from build123d import *

# Parameters (mm, degrees)
EXTRUDE_1_DEPTH     = 3
SKETCH_2_R          = 1.65
CUT_EXTRUDE_1_DEPTH = 10
SKETCH_3_R          = 1.65
CUT_EXTRUDE_2_DEPTH = 10
SKETCH_4_R          = 1.65
CUT_EXTRUDE_3_DEPTH = 10
SKETCH_5_R          = 1.65
CUT_EXTRUDE_4_DEPTH = 10
SKETCH_6_R          = 1.65
CUT_EXTRUDE_5_DEPTH = 10
SKETCH_7_R          = 1.65
CUT_EXTRUDE_6_DEPTH = 10
CUT_EXTRUDE_7_DEPTH = 10
FILLET_1_R          = 5


with BuildPart() as part:
    # 草图1 → 凸台-拉伸1 (new body)
    with BuildSketch(Plane.XY):
        with BuildLine():
            Line((-87.5, 103.859649123), (87.5, 103.859649123))
            ThreePointArc((87.5, 103.859649123), (91.035533906, 102.395183029), (92.5, 98.859649123))
            Line((92.5, 98.859649123), (92.5, -13.640350877))
            Line((92.5, -13.640350877), (50, -56.140350877))
            Line((50, -56.140350877), (-50, -56.140350877))
            Line((-50, -56.140350877), (-92.5, -13.640350877))
            Line((-92.5, -13.640350877), (-92.5, 98.859649123))
            ThreePointArc((-92.5, 98.859649123), (-91.035533906, 102.395183029), (-87.5, 103.859649123))
        make_face()
    extrude(amount=EXTRUDE_1_DEPTH)

    # 草图2 → 切除-拉伸1 (cut)
    with BuildSketch(Plane.XY.offset(3)):
        with Locations((-28.5, 95.359649123)):
            Circle(SKETCH_2_R)
        with Locations((28.5, 95.359649123)):
            Circle(SKETCH_2_R)
        with Locations((-28.5, 55.359649123)):
            Circle(SKETCH_2_R)
        with Locations((28.5, 55.359649123)):
            Circle(SKETCH_2_R)
    extrude(amount=-CUT_EXTRUDE_1_DEPTH, mode=Mode.SUBTRACT)

    # 草图3 → 切除-拉伸2 (cut)
    with BuildSketch(Plane.XY.offset(3)):
        with Locations((-87.5, 80.059649123)):
            Circle(SKETCH_3_R)
        with Locations((-45.5, 80.059649123)):
            Circle(SKETCH_3_R)
        with Locations((-87.5, 11.859649123)):
            Circle(SKETCH_3_R)
        with Locations((-45.5, 11.859649123)):
            Circle(SKETCH_3_R)
    extrude(amount=-CUT_EXTRUDE_2_DEPTH, mode=Mode.SUBTRACT)

    # 草图4 → 切除-拉伸3 (cut)
    with BuildSketch(Plane.XY.offset(3)):
        with Locations((42.5, 77.859649123)):
            Circle(SKETCH_4_R)
        with Locations((88.5, 77.859649123)):
            Circle(SKETCH_4_R)
        with Locations((42.5, 31.859649123)):
            Circle(SKETCH_4_R)
        with Locations((88.5, 31.859649123)):
            Circle(SKETCH_4_R)
    extrude(amount=-CUT_EXTRUDE_3_DEPTH, mode=Mode.SUBTRACT)

    # 草图5 → 切除-拉伸4 (cut)
    with BuildSketch(Plane.XY.offset(3)):
        with Locations((-39.3, 0.859649123)):
            Circle(SKETCH_5_R)
        with Locations((39.3, 0.859649123)):
            Circle(SKETCH_5_R)
        with Locations((-39.3, -51.140350877)):
            Circle(SKETCH_5_R)
        with Locations((39.3, -51.140350877)):
            Circle(SKETCH_5_R)
    extrude(amount=-CUT_EXTRUDE_4_DEPTH, mode=Mode.SUBTRACT)

    # 草图6 → 切除-拉伸5 (cut)
    with BuildSketch(Plane.XY.offset(3)):
        with Locations((-56.5, 98.359649123)):
            Circle(SKETCH_6_R)
        with Locations((56.5, 98.359649123)):
            Circle(SKETCH_6_R)
        with Locations((-45, -11.640350877)):
            Circle(SKETCH_6_R)
        with Locations((45, -11.640350877)):
            Circle(SKETCH_6_R)
    extrude(amount=-CUT_EXTRUDE_5_DEPTH, mode=Mode.SUBTRACT)

    # 草图7 → 切除-拉伸6 (cut)
    with BuildSketch(Plane.XY.offset(3)):
        with Locations((-13, 93.859649123)):
            Circle(SKETCH_7_R)
        with Locations((13, 93.859649123)):
            Circle(SKETCH_7_R)
        with Locations((13, 33.859649123)):
            Circle(SKETCH_7_R)
        with Locations((-13, 33.859649123)):
            Circle(SKETCH_7_R)
    extrude(amount=-CUT_EXTRUDE_6_DEPTH, mode=Mode.SUBTRACT)

    # 草图8 → 切除-拉伸7 (cut)
    with BuildSketch(Plane.XY.offset(3)):
        with BuildLine():
            Line((-20, 22.217358158), (20, 22.217358158))
            ThreePointArc((20, 22.217358158), (23.535533906, 20.752892063), (25, 17.217358158))
            Line((25, 17.217358158), (25, -22.782641842))
            ThreePointArc((25, -22.782641842), (23.535533906, -26.318175748), (20, -27.782641842))
            Line((20, -27.782641842), (-20, -27.782641842))
            ThreePointArc((-20, -27.782641842), (-23.535533906, -26.318175748), (-25, -22.782641842))
            Line((-25, -22.782641842), (-25, 17.217358158))
            ThreePointArc((-25, 17.217358158), (-23.535533906, 20.752892063), (-20, 22.217358158))
        make_face()
    extrude(amount=-CUT_EXTRUDE_7_DEPTH, mode=Mode.SUBTRACT)

    # 圆角1
    fillet_1_edges = [part.edges().sort_by_distance(p)[0] for p in [
        (-92.5, -13.640350877, 1.5),
        (92.5, -13.640350877, 1.5),
        (50, -56.140350877, 1.5),
        (-50, -56.140350877, 1.5),
    ]]
    fillet(fillet_1_edges, radius=FILLET_1_R)


solid = part.part
Source: CAD feature listing. Evaluate the final solid. Frame: model axes, mm. A direction names the side the tool comes from. Coordinates: 2 decimals unless noted, no trailing zeros. Loops run counter-clockwise (first coordinate to the right, second up) from the corner with the lowest first, then second, coordinate; pieces in that order, holes last. Notation, with made-up numbers: M 51.5,-37 L 109.5,-37 A19 cw 109.5,-21 Z; hole C 51,-4.5 d7. An arc over 180 degrees is marked long. Answer in a Markdown table with one row per item.
Q1. Ray query, probe 1 along Y at (x, z) = (-28.5, 2.3); probe 2 along Y at (x, z) = (-19.5, 2); probe 3 along Y at (x, z) = (39.3, 2). Return the intervals inside material, ascending. Write a range as from..to.
Answers below:
| item | result |
|---|---|
| probe 1 | y = -56.14..53.71, 57.01..93.71, 97.01..103.86 |
| probe 2 | y = -56.14..-27.78, 22.22..103.86 |
| probe 3 | y = -56.14..-52.79, -49.49..-0.79, 2.51..103.86 |
Q2. Draft query along X for faces 3 (the cylindrical face through (23.574, -26.279, 1.521)), 4 (the flat face through (1, 25, 3)), 5 (the flat face through (71.53, -34.61, 1.48)), 6 (the cylindrical face through (-91.07, 102.36, 1.48)). Return one class per face: pulls with the +X half, pulls with the -X half, needs draft (parallel to the pull), parting line crosses it, or undercut.
Answers below:
| item | result |
|---|---|
| face 3 | undercut |
| face 4 | needs draft |
| face 5 | pulls with the +X half |
| face 6 | pulls with the -X half |
Q3. Section A-A on x = 6. Return the cut outline in (y, z), plus the area to 3 significant figures.
Answers below:
| item | result |
|---|---|
| outline | M -56.14,0 L -27.78,0 L -27.78,3 L -56.14,3 Z; M 22.22,0 L 103.86,0 L 103.86,3 L 22.22,3 Z |
| area | 330 mm^2 |
Q4. Section B-B on z = 2.1. State how many separate pieces and enclosed holes the cut face has, plus the area to 3 significant figures.
Answers below:
| item | result |
|---|---|
| separate pieces | 1 |
| enclosed holes | 25 |
| area | 25,100 mm^2 |
Q5. Set-up query: faces 1 (the cylindrical face through (91, 102.43, 1.48)), 2 (the cylindrical face through (-23.496, -26.357, 1.521)). Return all of +Z, -Z, +X, -X, +Y, -Y with unobstructed straight access to the full face (end or side cutting, diameter ignored); none if empty.
Answers below:
| item | result |
|---|---|
| face 1 | +Z, -Z, +X, +Y |
| face 2 | +Z, -Z |
Q6. Section C-C on x = -65.5. Return the cut outline in (y, z).
Answers below:
| item | result |
|---|---|
| outline | M -40.64,0 L 103.86,0 L 103.86,3 L -40.64,3 Z |
Q7. First-contact query: pin 1 (4 mm diameter, centred on x = -87.5, y = 80.06, fed in from -Z). Flat tip, straight axial feed; report the tip coordinate or a pass-through.
Answers below:
| item | result |
|---|---|
| pin 1 | stops at z = 0 |
